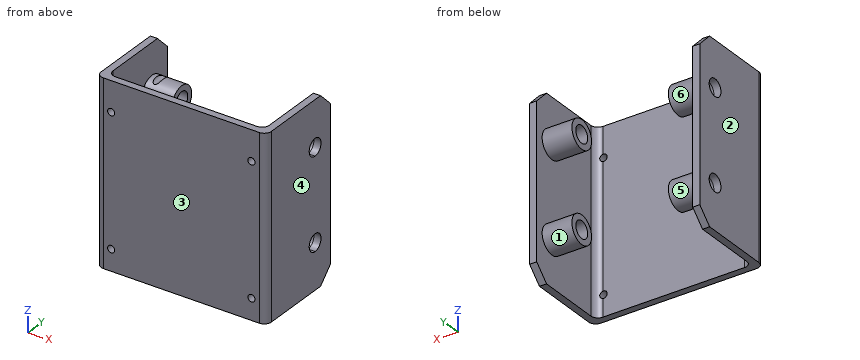
```python
from build123d import *

# Parameters (mm, degrees)
BOSS_EXTRUDE1_DEPTH     = 128
FILLET1_R               = 5
CHAMFER1_SIZE           = 10
SKETCH3_R               = 6
CUT_EXTRUDE1_DEPTH      = 121
SKETCH5_R               = 10
BOSS_EXTRUDE2_DEPTH     = 21
SKETCH6_R               = 10
BOSS_EXTRUDE3_DEPTH     = 21
SKETCH7_R               = 6
CUT_EXTRUDE2_DEPTH      = 6
CUT_EXTRUDE2_DEPTH_BACK = 116
SKETCH8_R               = 2.5
CUT_EXTRUDE3_DEPTH      = 66


with BuildPart() as part:
    # Sketch2 → Boss-Extrude1 (new body)
    with BuildSketch(Plane.XY):
        Polygon((-55, 30), (-55, -30), (55, -30), (55, 30), (60, 30), (60, -35), (-60, -35), (-60, 30), align=None)
    extrude(amount=BOSS_EXTRUDE1_DEPTH)

    # Fillet1
    fillet1_edges = [part.edges().sort_by_distance(p)[0] for p in [
        (60, -35, 64),
        (-60, -35, 64),
        (-55, -30, 64),
        (55, -30, 64),
    ]]
    fillet(fillet1_edges, radius=FILLET1_R)

    # Chamfer1
    chamfer1_edges = [part.edges().sort_by_distance(p)[0] for p in [
        (-57.5, 30, 128),
        (57.5, 30, 128),
        (57.5, 30, 0),
        (-57.5, 30, 0),
    ]]
    chamfer(chamfer1_edges, length=CHAMFER1_SIZE)

    # Sketch3 → Cut-Extrude1 (cut, through all)
    with BuildSketch(Plane(origin=(60, 0, 0), x_dir=(0, 0, -1), z_dir=(1, 0, 0))):
        with Locations((-96, 14.48521638)):
            Circle(SKETCH3_R)
        with Locations((-32, 14.48521638)):
            Circle(SKETCH3_R)
    extrude(amount=-CUT_EXTRUDE1_DEPTH, mode=Mode.SUBTRACT)

    # Sketch5 → Boss-Extrude2 (add)
    with BuildSketch(Plane.ZY.offset(-55)):
        with Locations((32, 14.48521638)):
            Circle(SKETCH5_R)
        with Locations((96, 14.48521638)):
            Circle(SKETCH5_R)
    extrude(amount=BOSS_EXTRUDE2_DEPTH)

    # Sketch6 → Boss-Extrude3 (add)
    with BuildSketch(Plane(origin=(-55, 0, 0), x_dir=(0, 0, -1), z_dir=(1, 0, 0))):
        with Locations((-32, 14.48521638)):
            Circle(SKETCH6_R)
        with Locations((-96, 14.48521638)):
            Circle(SKETCH6_R)
    extrude(amount=BOSS_EXTRUDE3_DEPTH)

    # Sketch7 → Cut-Extrude2 (cut, two sides)
    with BuildSketch(Plane.ZY.offset(55)) as cut_extrude2_sk:
        with Locations((32, 14.48521638)):
            Circle(SKETCH7_R)
        with Locations((96, 14.48521638)):
            Circle(SKETCH7_R)
    extrude(amount=CUT_EXTRUDE2_DEPTH, mode=Mode.SUBTRACT)
    extrude(cut_extrude2_sk.sketch, amount=-CUT_EXTRUDE2_DEPTH_BACK, mode=Mode.SUBTRACT)

    # Sketch8 → Cut-Extrude3 (cut, through all)
    with BuildSketch(Plane.XZ.offset(35)):
        with Locations((49.450316968, 14.929077734)):
            Circle(SKETCH8_R)
        with Locations((-49.450316968, 14.929077734)):
            Circle(SKETCH8_R)
        with Locations((-49.450316968, 106.821296535)):
            Circle(SKETCH8_R)
        with Locations((49.450316968, 106.821296535)):
            Circle(SKETCH8_R)
    extrude(amount=-CUT_EXTRUDE3_DEPTH, mode=Mode.SUBTRACT)


solid = part.part
```
The listing builds one solid part. Answer for the finished solid, in the listing's coordinates (mm). Face numbers are marked on the shaded views. A direction names the side the tool comes from. Give positions to 0.01 mm unless a question says otherwise; leave off trailing zeros. Order: outer loops, then holes, each group sorted by start corner. A loop starts at its lowest first (then second) coordinate and runs counter-clockwise, first axis right, second up.
Item 1: The part is cut by section A-A, the plane z = 32. Give the vertices of the cut face in (x, y), and give its area (3 significant figures).
From the geometry:
outline: (-60, -30) arc R5 ccw to (-55, -35) - (55, -35) arc R5 ccw to (60, -30) - (60, 8.49) - (34, 8.49) - (34, 4.49) - (55, 4.49) - (55, -25) arc R5 cw to (50, -30) - (-50, -30) arc R5 cw to (-55, -25) - (-55, 4.49) - (-34, 4.49) - (-34, 8.49) - (-60, 8.49) - close; (-60, 20.49) - (-34, 20.49) - (-34, 24.49) - (-55, 24.49) - (-55, 30) - (-60, 30) - close; (34, 20.49) - (60, 20.49) - (60, 30) - (55, 30) - (55, 24.49) - (34, 24.49) - close
area: 1,420 mm2
Item 2: Find the intervals of material crossed by probe 1 along Y at (x, z) = (40, 96); probe 2 along X at (y, z) = (18, 48); probe 3 along Z at (x, y) = (-46.5, 15), in increasing order.
From the geometry:
probe 1: y = -35 to -30, 4.49 to 8.49, 20.49 to 24.49
probe 2: x = -60 to -55, 55 to 60
probe 3: z = 22.01 to 26.02, 37.98 to 41.99, 86.01 to 90.02, 101.98 to 105.99
Item 3: The part is cut by section C-C, the plane y = -18. Give the vertices of the cut face in (x, z).
From the geometry:
outline: (-60, 0) - (-55, 0) - (-55, 128) - (-60, 128) - close; (55, 0) - (60, 0) - (60, 128) - (55, 128) - close
Item 4: The part is cut by section D-D, the plane z = 70. Give the vertices of the cut face in (x, y), and give its area (3 significant figures).
From the geometry:
outline: (-60, -30) arc R5 ccw to (-55, -35) - (55, -35) arc R5 ccw to (60, -30) - (60, 30) - (55, 30) - (55, -25) arc R5 cw to (50, -30) - (-50, -30) arc R5 cw to (-55, -25) - (-55, 30) - (-60, 30) - close
area: 1,200 mm2
Item 5: Which of the six approach directions +Z, -Z, +X, -X, +Y, -Y give full straight-line access (tool end or side, diameter ignored) to the marked faces 1 and 2?
From the geometry:
face 1: none
face 2: +Z, -Z, -X, +Y, -Y
Item 6: Given pin 1 Ø2 at (x, z) = (5.5, 100.5) entering from +Y; pin 2 Ø4 at (x, y) = (-33.5, 17.5) entering from -Z; pin 3 Ø6.5 at (x, z) = (49.45, 14.93) entering from +Y, each flat-ended and moving along its own axis, determine where each tip first touches the part or whether it passes through.
From the geometry:
pin 1: stops at y = -30
pin 2: stops at z = 22.06
pin 3: stops at y = -29.21
Item 7: For a pull along Y with two mould halves and no side action, classify the marked faces 3, 4, 5 and 6 as pulls with the +Y half, pulls with the -Y half, needs draft (parallel to the pull), parting line crosses it, or undercut.
From the geometry:
face 3: pulls with the -Y half
face 4: needs draft
face 5: undercut
face 6: undercut
Item 8: The part is cut by section B-B, the plane x = -37. Give the vertices of the cut face in (y, z), and give its area (3 significant figures).
From the geometry:
outline: (-35, 0) - (-30, 0) - (-30, 128) - (-35, 128) - close; circle Ø20 at (14.49, 32); circle Ø20 at (14.49, 96); hole circle Ø12 at (14.49, 32); hole circle Ø12 at (14.49, 96)
area: 1,040 mm2
